Can you work these out from the model? Positions are in its coordinate system, mm. A direction names the side the tool comes from. Round coordinates to 2 decimals unless told otherwise and drop trailing zeros. Write each loop counter-clockwise with the first axis right and the second up, starting at its lowest first coordinate (ties: lowest second). Pieces come first, ordered by that corner, then holes. Notation, with made-up numbers: (84.25, 43) -> (129.25, 43) arc R17 ccw to (129.25, 62) -> close; hole circle Ø9 at (45, 44). An arc over 180 degrees is marked (long way). Use CSV: the item, a comma, the result in double quotes.
```python
from build123d import *

# Parameters (mm, degrees)
SKETCH1_W                   = 55.5
SKETCH1_H                   = 38.2
BRACKETBASE_DEPTH           = 2.5
SKETCH2_W                   = 7
SKETCH2_H                   = 20.5
SERVOMOUNTINGHOLETABS_DEPTH = 2.5
SKETCH3_R                   = 2
SERVOMOUNTINGHOLES_DEPTH    = 2.5
SKETCH4_W                   = 55.5
SKETCH4_H                   = 2.5
BASEWALL_DEPTH              = 23
SKETCH5_R                   = 2.125
M4MOUNTINGHOLE_DEPTH        = 2.5
SKETCH6_R                   = 5.7
BASETRIM_DEPTH              = 2.5
FILLET1_R                   = 2
SKETCH7_R                   = 2.125
CUT_EXTRUDE1_DEPTH          = 10
BOSS_EXTRUDE1_START         = -2.5
SKETCH8_R                   = 2.125
BOSS_EXTRUDE1_DEPTH         = 2.5


with BuildPart() as part:
    # Sketch1 → bracketBase (new body)
    with BuildSketch(Plane(origin=(0, 0, 0), x_dir=(1, 0, 0), z_dir=(0, 1, 0))):
        with Locations((27.75, 19.1)):
            Rectangle(SKETCH1_W, SKETCH1_H)
    extrude(amount=BRACKETBASE_DEPTH)

    # Sketch2 → servoMountingHoleTabs (add)
    with BuildSketch(Plane.XY.offset(-8.2)):
        with Locations((3.5, 12.75)):
            Rectangle(SKETCH2_W, SKETCH2_H)
        with Locations((52, 12.75)):
            Rectangle(SKETCH2_W, SKETCH2_H)
    extrude(amount=SERVOMOUNTINGHOLETABS_DEPTH)

    # Sketch3 → servoMountingHoles (cut)
    with BuildSketch(Plane.XY.offset(-5.7)):
        with Locations((3.75, 17.75)):
            Circle(SKETCH3_R)
        with Locations(Location((3.75, 7.75, 0), (0, 0, 180))):
            Circle(SKETCH3_R)
        with Locations((51.75, 7.75)):
            Circle(SKETCH3_R)
        with Locations(Location((51.75, 17.75, 0), (0, 0, 180))):
            Circle(SKETCH3_R)
    extrude(amount=-SERVOMOUNTINGHOLES_DEPTH, mode=Mode.SUBTRACT)

    # Sketch4 → baseWall (add)
    with BuildSketch(Plane(origin=(0, 0, 0), x_dir=(1, 0, 0), z_dir=(0, 1, 0))):
        with Locations((27.75, 39.45)):
            Rectangle(SKETCH4_W, SKETCH4_H)
    extrude(amount=BASEWALL_DEPTH)

    # Sketch5 → M4mountingHole (cut)
    with BuildSketch(Plane.XY.offset(-38.2)):
        with Locations((38.25, 12.75)):
            Circle(SKETCH5_R)
    extrude(amount=-M4MOUNTINGHOLE_DEPTH, mode=Mode.SUBTRACT)

    # Sketch6 → baseTrim (cut)
    with BuildSketch(Plane(origin=(0, 2.5, 0), x_dir=(1, 0, 0), z_dir=(0, 1, 0))):
        Circle(SKETCH6_R)
        with Locations((55.5, 0)):
            Circle(SKETCH6_R)
    extrude(amount=-BASETRIM_DEPTH, mode=Mode.SUBTRACT)

    # Fillet1
    fillet1_edges = [part.edges().sort_by_distance(p)[0] for p in [
        (0, 23, -6.95),
        (7, 23, -6.95),
        (55.5, 23, -6.95),
        (48.5, 23, -6.95),
        (55.5, 23, -39.45),
        (0, 23, -39.45),
    ]]
    fillet(fillet1_edges, radius=FILLET1_R)

    # Sketch7 → Cut-Extrude1 (cut)
    with BuildSketch(Plane(origin=(0, 0, -40.7), x_dir=(-1, 0, 0), z_dir=(0, 0, -1))):
        with Locations((-17.25, 12.75)):
            Circle(SKETCH7_R)
    extrude(amount=-CUT_EXTRUDE1_DEPTH, mode=Mode.SUBTRACT)

    # Sketch8 → Boss-Extrude1 (add)
    with BuildSketch(Plane.XY.offset(-38.2).offset(BOSS_EXTRUDE1_START)):
        with Locations((17.25, 12.75)):
            Circle(SKETCH8_R)
    extrude(amount=BOSS_EXTRUDE1_DEPTH)


solid = part.part
```
Q1. On a 3-axis mill with a long thin cutter (end or side, diameter ignored), from which of +Z, -Z, +X, -X, +Y, -Y can I reach the whole of each face in a straight line? I mean faces 4 (the face through (6.4, 22.43, -6.93)), 5 (the face through (52.01, 15.767, -6.932)), 6 (the face through (27, 13, -38.2)). Say none if no direction works.
Resolved:
face 4,"+Z, +Y"
face 5,"+Z"
face 6,"+X, -X, +Y"
Q2. Suppose I cut it at A-A (y = 12.75). Write out the boundary of the cut face in (x, z) (3 decimals), and give its area (3 significant figures).
Resolved:
outline,"(0, -40.7) -> (36.125, -40.7) -> (36.125, -38.2) -> (0, -38.2) -> close; (0, -8.2) -> (7, -8.2) -> (7, -5.7) -> (0, -5.7) -> close; (40.375, -40.7) -> (55.5, -40.7) -> (55.5, -38.2) -> (40.375, -38.2) -> close; (48.5, -8.2) -> (55.5, -8.2) -> (55.5, -5.7) -> (48.5, -5.7) -> close"
area,"163 mm^2"
Q3. Suppose I cut it at C-C (y = 7.75). Write out the boundary of the cut face in (x, z), and give its area (3 significant figures).
Resolved:
outline,"(0, -40.7) -> (55.5, -40.7) -> (55.5, -38.2) -> (0, -38.2) -> close; (0, -8.2) -> (1.75, -8.2) -> (1.75, -5.7) -> (0, -5.7) -> close; (5.75, -8.2) -> (7, -8.2) -> (7, -5.7) -> (5.75, -5.7) -> close; (48.5, -8.2) -> (49.75, -8.2) -> (49.75, -5.7) -> (48.5, -5.7) -> close; (53.75, -8.2) -> (55.5, -8.2) -> (55.5, -5.7) -> (53.75, -5.7) -> close"
area,"154 mm^2"
Q4. Please list where these lines run through material, in increasing order: probe 1 along Y at (x, z) = (51.75, -7.3); probe 2 along Z at (x, y) = (6, 12); probe 3 along Y at (x, z) = (43, -10).
Resolved:
probe 1,"y = 0 to 5.75, 9.75 to 15.75, 19.75 to 23"
probe 2,"z = -40.7 to -38.2, -8.2 to -5.7"
probe 3,"y = 0 to 2.5"
Q5. Suppose I cut it at D-D (x = 51.75). Write out the boundary of the cut face in (y, z), and give its area (3 significant figures).
Resolved:
outline,"(0, -40.7) -> (23, -40.7) -> (23, -38.2) -> (2.5, -38.2) -> (2.5, -8.2) -> (5.75, -8.2) -> (5.75, -5.7) -> (2.5, -5.7) -> (2.5, -4.29) -> (0, -4.29) -> close; (9.75, -8.2) -> (15.75, -8.2) -> (15.75, -5.7) -> (9.75, -5.7) -> close; (19.75, -8.2) -> (23, -8.2) -> (23, -5.7) -> (19.75, -5.7) -> close"
area,"174 mm^2"
Q6. If we mould it in two halves opening along X, with no side actions, what happens to faces 1 (the face through (27, 23, -39)), 2 (the face through (54.9, 22.43, -39.47)), 3 (the face through (7, 12, -7))? For each: released by +X, released by -X, zero draft, split by the parting line, or undercut.
Resolved:
face 1,"zero draft"
face 2,"released by +X"
face 3,"undercut"
Q7. Suppose I cut it at B-B (x = 38.25). Write out the boundary of the cut face in (y, z) (3 decimals), and give its area (3 significant figures).
Resolved:
outline,"(0, -40.7) -> (10.625, -40.7) -> (10.625, -38.2) -> (2.5, -38.2) -> (2.5, 0) -> (0, 0) -> close; (14.875, -40.7) -> (23, -40.7) -> (23, -38.2) -> (14.875, -38.2) -> close"
area,"142 mm^2"
Q8. Will these pins go through, and if not, where does the flat tip stop? P1, Ø3, axis at x = 3.75, y = 17.75, coming from the +Z side; P2, Ø19, axis at x = 40, z = -18, coming from the +Y side; P3, Ø7.5, axis at x = 2, y = 10, coming from the +Z side.
Resolved:
P1,"stops at z = -38.2"
P2,"stops at y = 2.5"
P3,"stops at z = -5.7"
